Geometry: final body of the model. Coordinates: model frame, mm. A direction names the side the tool comes from. Give positions to 0.01 mm unless a question says otherwise; leave off trailing zeros. Loops run counter-clockwise (first coordinate to the right, second up) from the corner with the lowest first, then second, coordinate; pieces in that order, holes last. Notation, with made-up numbers: (8, 17) - (66, 17) arc R19 ccw to (66, 36) - close; hole circle Ø2 at (53.25, 23.25). An arc over 180 degrees is marked (long way). Use one line per item in the form item = value.
```python
from build123d import *

# Parameters (mm, degrees)
PAD_DEPTH          = 0.6
POLARPATTERN_COUNT = 5


with BuildPart() as part:
    # Sketch → Revolution (revolve)
    with BuildSketch(Plane.XZ):
        with BuildLine():
            Line((16, 0), (16, 2))
            ThreePointArc((16, 2), (13.071068, 9.071068), (6, 12))
            Line((3.8, 12), (6, 12))
            Line((3.8, 8), (3.8, 12))
            Line((1.8, 6), (3.8, 8))
            Line((1.8, 6), (1.8, 0))
            Line((1.8, 0), (3.8, 0))
            Line((3.8, 0), (3.8, 5.5))
            Line((3.8, 5.5), (5.5, 7.2))
            Line((5.5, 7.2), (5.5, 10))
            ThreePointArc((14, 2), (11.478291, 7.836309), (5.5, 10))
            Line((14, 0), (14, 2))
            Line((16, 0), (14, 0))
        make_face()
    revolve(axis=Axis((0, 0, 0), (0, 0, 1)))

    # Sketch001 → Pad (new body, symmetric)
    with BuildSketch(Plane.XZ):
        with BuildLine():
            Line((14.5, 0), (14.5, 2))
            ThreePointArc((14.5, 2), (11.892744, 8.543126), (5.5, 11.5))
            Line((5.5, 7.5), (5.5, 11.5))
            Line((3.5, 5.5), (5.5, 7.5))
            Line((3.5, 0), (3.5, 5.5))
            Line((3.5, 0), (14.5, 0))
        make_face()
    pad = extrude(amount=PAD_DEPTH, both=True)

    # PolarPattern: Pad ×5 about axis
    polarpattern_axis = Axis((0, 0, 0), (0, 0, 1))
    for i in range(1, POLARPATTERN_COUNT):
        add(pad.rotate(polarpattern_axis, i * 360 / POLARPATTERN_COUNT))


solid = part.part
```
(1) Pin query (flat end, axial travel): P1, Ø4, axis at x = 0, y = 0, coming from the +Z side; P2, Ø5, axis at y = -7, z = 10.5, coming from the +X side; P3, Ø4, axis at y = 0.5, z = 10.5, coming from the -X side. Return the tip coordinate at first contact, or that it passes through.
Solution:
P1 = 6.2
P2 = 12.48
P3 = -13.59
(2) Material intervals for L1, parallel to X at y = 11.5, z = 2; L2, parallel to Y at x = -6, z = 1; L3, parallel to X at y = 7, z = 2.5, sorted ascending. Write a range as from..to.
Solution:
L1 = -11.12..-7.98, 3.11..4.37, 7.98..11.12
L2 = -14.83..-12.65, -5.1..-3.62, 3.62..5.1, 12.65..14.83
L3 = -14.37..-12.11, -10.66..-8.61, 1.64..2.91, 12.11..14.37
(3) Access query for faces 4 (the face through (-1.654, 5.246, 8.62)), 5 (the face through (3.1, 2.2, 2.8)), 6 (the face through (-3.47, -15.62, 1.01)). Directions: +Z, -Z, +X, -X, +Y, -Y. A direction counts if a zero-diameter tool reaches every point of the face in a straight line with its end or side. Return the directions, or none.
Solution:
face_4 = none
face_5 = -Z
face_6 = +Z, -Z
(4) Pull-direction query (Z, two-part tool) for faces 1 (the face through (9, 0.6, 4)), 2 (the face through (-1.746, -5.216, 8.62)), 3 (the face through (-1.41, -4.24, 6.17)); classes: released by +Z, released by -Z, zero draft, split by the parting line, or undercut.
Solution:
face_1 = zero draft
face_2 = undercut
face_3 = released by -Z
(5) Cut plane B-B (z = 3.25). Give the number of separate pieces and of enclosed holes in the cut face, plus the area to 3 significant figures.
Solution:
separate_pieces = 1
enclosed_holes = 6
area = 285 mm2
(6) Cut plane A-A (z = 1.25). Return the cut outline in (x, y), plus the area to 3 significant figures.
Solution:
outline = circle Ø32 at (0, 0); hole (-11.67, -7.74) - (-3.39, -1.72) arc R3.8 cw to (-3.39, 1.72) - (-11.67, 7.74) arc R14 ccw to start; hole (-10.96, -8.71) arc R14 ccw to (3.75, -13.49) - (0.59, -3.75) arc R3.8 cw to (-2.68, -2.69) - close; hole (-10.96, 8.71) - (-2.68, 2.69) arc R3.8 cw to (0.59, 3.75) - (3.75, 13.49) arc R14 ccw to start; hole circle Ø3.6 at (0, 0); hole (1.73, -3.38) - (4.89, -13.12) arc R14 ccw to (13.99, -0.6) - (3.75, -0.6) arc R3.8 cw to start; hole (1.73, 3.38) arc R3.8 cw to (3.75, 0.6) - (13.99, 0.6) arc R14 ccw to (4.89, 13.12) - close
area = 285 mm2
